Can you work these out from the model? Positions are in its coordinate system, mm. A direction names the side the tool comes from. Give positions to 0.01 mm unless a question says otherwise; leave off trailing zeros. Loops run counter-clockwise (first coordinate to the right, second up) from the corner with the lowest first, then second, coordinate; pieces in that order, holes last. Notation, with made-up numbers: (-33, 3.5) - (-28, 3.5) arc R14 ccw to (-28, 11.5) - close; hole circle Ø1 at (62, -13). An arc over 180 degrees is marked (long way). Answer in a Markdown table with one row per item.
from build123d import *

# Parameters (mm, degrees)
SKETCH1_R                = 1.143
SKETCH1_R_2              = 0.75
BOSS_EXTRUDE1_DEPTH      = 1.651
SKETCH2_W                = 10.16
SKETCH2_H                = 5.08
BOSS_EXTRUDE2_DEPTH      = 1.651
BOSS_EXTRUDE2_DEPTH_BACK = 1.651


with BuildPart() as part:
    # Sketch1 → Boss-Extrude1 (new body)
    with BuildSketch(Plane(origin=(0, 0, 0), x_dir=(1, 0, 0), z_dir=(0, 1, 0))):
        with BuildLine():
            Line((0, 6.096), (0, 0))
            Line((0, 0), (45.974, 0))
            Line((45.974, 0), (45.974, 3.175))
            Line((45.974, 3.175), (44.7675, 3.175))
            ThreePointArc((44.7675, 3.175), (43.942, 4.0005), (44.7675, 4.826))
            Line((44.7675, 4.826), (45.974, 4.826))
            Line((45.974, 4.826), (45.974, 6.731))
            Line((45.974, 6.731), (19.812, 6.731))
            Line((19.812, 6.731), (19.812, 1.651))
            Line((19.812, 1.651), (9.652, 1.651))
            Line((9.652, 1.651), (9.652, 6.731))
            Line((9.652, 6.731), (7.112, 6.731))
            Line((7.112, 6.731), (7.112, 6.096))
            Line((7.112, 6.096), (0, 6.096))
        make_face()
        with Locations((2.159, 3.2258)):
            Circle(SKETCH1_R, mode=Mode.SUBTRACT)
        with Locations((30.0228, 3.302)):
            Circle(SKETCH1_R, mode=Mode.SUBTRACT)
        with Locations((6.6936, 4.1282)):
            Circle(SKETCH1_R_2, mode=Mode.SUBTRACT)
    extrude(amount=BOSS_EXTRUDE1_DEPTH)

    # Sketch2 → Boss-Extrude2 (add, two sides)
    with BuildSketch(Plane(origin=(0, 1.651, 0), x_dir=(1, 0, 0), z_dir=(0, 1, 0))) as boss_extrude2_sk:
        with Locations((14.732, 4.191)):
            Rectangle(SKETCH2_W, SKETCH2_H)
    extrude(amount=BOSS_EXTRUDE2_DEPTH)
    extrude(boss_extrude2_sk.sketch, amount=-BOSS_EXTRUDE2_DEPTH_BACK)


solid = part.part
Q1. For pin 1 (1.3 mm diameter, centred on x = 45.5, y = 0.5, fed in from +Z); pin 2 (1.8 mm diameter, centred on x = 3.5, y = 0.5, fed in from -Z); pin 3 (1.3 mm diameter, centred on y = 3, z = -4.5, fed in from +X); pin 4 (0.8 mm diameter, centred on y = 3, z = -3.5, fed in from -X), each with a flat end and sliding along its axis, tell me the tip position at first contact or that it passes through.
Checked values:
| item | result |
|---|---|
| pin 1 | stops at z = 0 |
| pin 2 | stops at z = -6.1 |
| pin 3 | stops at x = 19.81 |
| pin 4 | stops at x = 9.65 |
Q2. If we mould it in two halves opening along X, with no side actions, what happens to faces 6 (the face through (22, 1, -6.731)), 7 (the face through (2.01, 0.81, -4.36)), 8 (the face through (9.652, 2, -4))? For each: released by +X, released by -X, zero draft, split by the parting line, or undercut.
Checked values:
| item | result |
|---|---|
| face 6 | zero draft |
| face 7 | undercut |
| face 8 | released by -X |
Q3. Imagine slicing it at D-D, the plane y = 2.55. Write out the boundary of the cut face in (x, z).
Checked values:
| item | result |
|---|---|
| outline | (9.65, -6.73) - (19.81, -6.73) - (19.81, -1.65) - (9.65, -1.65) - close |
Q4. Imagine slicing it at C-C, the plane x = 12.5. Write out the boundary of the cut face in (y, z), and give its area (3 significant figures).
Checked values:
| item | result |
|---|---|
| outline | (0, -6.73) - (3.3, -6.73) - (3.3, -1.65) - (1.65, -1.65) - (1.65, 0) - (0, 0) - close |
| area | 19.5 mm² |
Q5. Imagine slicing it at A-A, the plane z = -5.5. Write out the boundary of the cut face in (x, y), and give its area (3 significant figures).
Checked values:
| item | result |
|---|---|
| outline | (0, 0) - (45.97, 0) - (45.97, 1.65) - (19.81, 1.65) - (19.81, 3.3) - (9.65, 3.3) - (9.65, 1.65) - (0, 1.65) - close |
| area | 92.7 mm² |
Q6. Imagine slicing it at B-B, the plane y = 0.45. Count the separate pieces of the cut face and the enclosed holes in it, and give its area (3 significant figures).
Checked values:
| item | result |
|---|---|
| separate pieces | 1 |
| enclosed holes | 3 |
| area | 292 mm² |
Q7. On a 3-axis mill with a long thin cutter (end or side, diameter ignored), from which of +Z, -Z, +X, -X, +Y, -Y can I reach the whole of each face in a straight line? I mean faces 1 (the face through (15, 2, -1.651)), 2 (the face through (4, 1, -6.096)), 3 (the face through (19.812, 2, -4)), 4 (the face through (45, 1, -4.826)), 5 (the face through (45.974, 1, -6)). Say none if no direction works.
Checked values:
| item | result |
|---|---|
| face 1 | +Z, +X, -X, +Y |
| face 2 | -Z, -X, +Y, -Y |
| face 3 | +Z, -Z, +X, +Y |
| face 4 | +X, +Y, -Y |
| face 5 | +Z, -Z, +X, +Y, -Y |
Q8. If I drill on line 1 (X direction, y = 1.25, z = -2.5); line 2 (Z direction, x = 19, y = 1.7); line 3 (Y direction, x = 5.5, z = -3.5), over which ranges is the centre line in solid material (lowest first)? Write a range as [from, to].
Checked values:
| item | result |
|---|---|
| line 1 | x = [0, 1.28], [3.04, 29.21], [30.84, 45.97] |
| line 2 | z = [-6.73, -1.65] |
| line 3 | y = [0, 1.65] |
